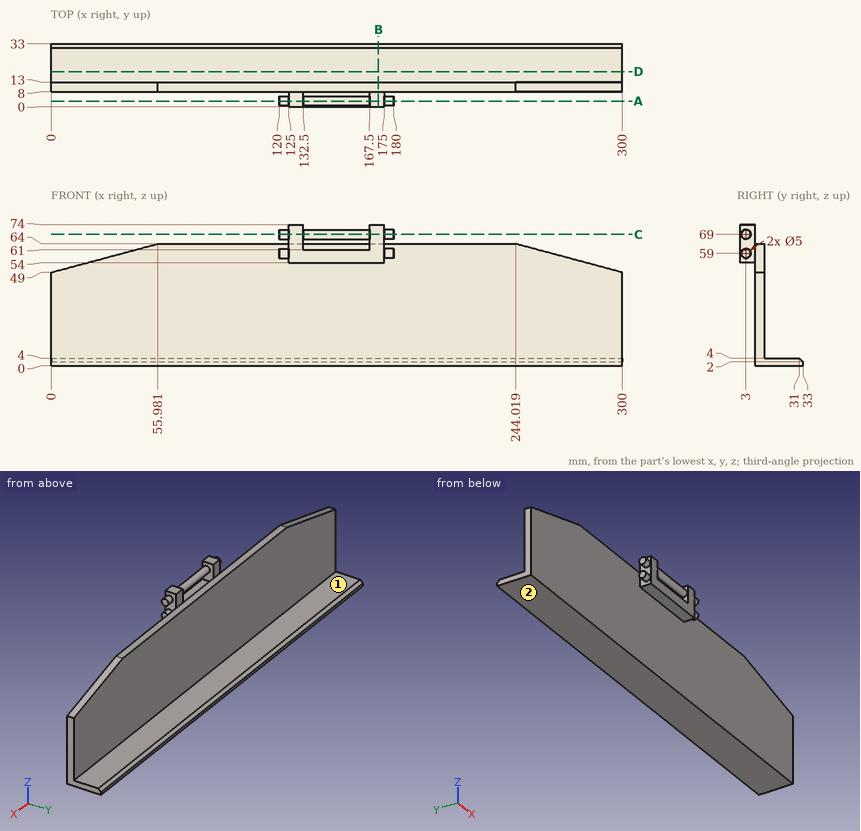
Print and shaded views of the part. All mm, measured from the part's lowest x, y and z. A direction names the side the tool comes from. Round coordinates to 2 decimals unless told otherwise and drop trailing zeros. Write each loop counter-clockwise with the first axis right and the second up, starting at its lowest first coordinate (ties: lowest second). Pieces come first, ordered by that corner, then holes. Notation, with made-up numbers: (89, 18) - (136, 18) arc R23 cw to (136, 52) - close; hole circle Ø11 at (50, -28.75). An arc over 180 degrees is marked (long way). Write each question's results on one line, items separated by ' | '. Start each with the question number.
Item 1: Which spindle directions (+Z, -Z, +X, -X, +Y, -Y) get a long thin tool onto all of the face, cutting with end or side? Do the marked faces 1 and 2. Say none if no direction does.
Item 2: Saw through at A-A (y = 3). Write the cut outline in (x, z).
Item 3: Saw through at B-B (x = 172). Write the cut outline in (y, z).
Item 4: Wall check: L1, parallel to Z at x = 178.5, y = 3.5; L2, parallel to Z at x = 107.5, y = 15; L3, parallel to Z at x = 28, y = 10. Give the ranges that are in metal, low to high. Write a range as [from, to].
Item 5: Saw through at D-D (y = 18.5). Write the cut outline in (x, z).
Item 6: Saw through at C-C (z = 69). Write the cut outline in (x, y).
Item 7: Drop flat-ended pins along their axis: P1, Ø3, axis at x = 161.5, z = 36.5, coming from the +Y side; P2, Ø2, axis at x = 130.5, z = 69.5, coming from the +Y side; P3, Ø4, axis at y = 2.5, z = 58.5, coming from the -X side. Give the stop position or say it passes through.
Results are:
1) face 1: +Z, +X, -X, +Y | face 2: -Z, +X, -X, +Y, -Y
2) outline: (120, 56.5) - (125, 56.5) - (125, 54) - (175, 54) - (175, 56.5) - (180, 56.5) - (180, 61.5) - (175, 61.5) - (175, 66.5) - (180, 66.5) - (180, 71.5) - (175, 71.5) - (175, 74) - (167.5, 74) - (167.5, 71.5) - (132.5, 71.5) - (132.5, 74) - (125, 74) - (125, 71.5) - (120, 71.5) - (120, 66.5) - (125, 66.5) - (125, 61.5) - (120, 61.5) - close; hole (132.5, 61) - (167.5, 61) - (167.5, 66.5) - (132.5, 66.5) - close
3) outline: (0, 54) - (8, 54) - (8, 0) - (33, 0) - (33, 2) - (31, 4) - (13, 4) - (13, 64) - (8, 64) - (8, 74) - (0, 74) - close
4) L1: z = [56.55, 61.45], [66.55, 71.45] | L2: z = [0, 4] | L3: z = [0, 56.5]
5) outline: (0, 0) - (300, 0) - (300, 4) - (0, 4) - close
6) outline: (120, 0.5) - (125, 0.5) - (125, 0) - (132.5, 0) - (132.5, 0.5) - (167.5, 0.5) - (167.5, 0) - (175, 0) - (175, 0.5) - (180, 0.5) - (180, 5.5) - (175, 5.5) - (175, 8) - (167.5, 8) - (167.5, 5.5) - (132.5, 5.5) - (132.5, 8) - (125, 8) - (125, 5.5) - (120, 5.5) - close
7) P1: stops at y = 13 | P2: stops at y = 8 | P3: stops at x = 120
